For this review, take the finished solid that the model builds, in its own axes (mm). Face numbers are marked on the shaded views. A direction names the side the tool comes from. Round coordinates to 2 decimals unless told otherwise and drop trailing zeros. Loops run counter-clockwise (first coordinate to the right, second up) from the corner with the lowest first, then second, coordinate; pieces in that order, holes last.
1. Clearance check with flat-ended pins moving along their axes: pin 1 Ø2 at (x, z) = (16, 13) entering from +Y; pin 2 Ø2 at (x, y) = (14, 8.5) entering from +Z; pin 3 Ø1.8 at (x, z) = (9.5, 6) entering from +Y. State where each tip first meets the part, or that it passes through.
2. Tool access review of the marked faces 4, 5 and 6: name each direction out of +Z, -Z, +X, -X, +Y, -Y from which nothing blocks a thin tool from reaching the whole face with its end or side.
3. Consider section A-A on y = 15. State the section outline as (x, z) points, then the cut area to 3 significant figures.
4. Consider section B-B on x = 10. State the section outline as (y, z) points, then the cut area to 3 significant figures.
5. Draft analysis for pull direction X (two halves, no side actions). For the marked faces 1, 2 and 3, state which applies: released by +X, released by -X, zero draft, split by the parting line, or undercut.
6. Consider section D-D on z = 13. State the section outline as (x, y) points.
7. Consider section C-C on x = 5.25. State the section outline as (y, z) points, then the cut area to 3 significant figures.
8. To check wall thickness, follow line 1 along Y through (x, z) = (10, 2.05); line 2 along Z through (x, y) = (6.75, 8); line 3 along Z through (x, y) = (3, 17.5). State the ranges of each line that lie inside material, in increasing order.
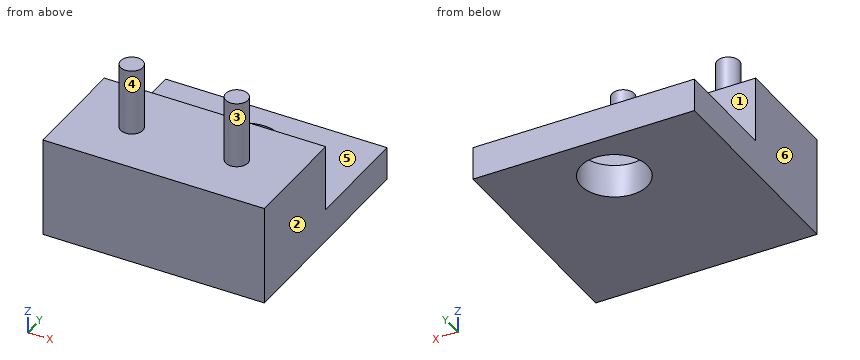
from build123d import *

# Parameters (mm, degrees)
SKETCH_1_W          = 20
SKETCH_1_H          = 20
EXTRUDE_1_DEPTH     = 9
SKETCH_2_R          = 1
EXTRUDE_2_DEPTH     = 6
SKETCH_3_W          = 20
SKETCH_3_H          = 10
CUT_EXTRUDE_1_DEPTH = 6
CUT_EXTRUDE_2_REACH = 32.725
SKETCH_4_R          = 3


with BuildPart() as part:
    # 草图1 → 凸台-拉伸1 (new body)
    with BuildSketch(Plane.XY):
        with Locations((10, 10)):
            Rectangle(SKETCH_1_W, SKETCH_1_H)
    extrude(amount=EXTRUDE_1_DEPTH)

    # 草图2 → 凸台-拉伸2 (add)
    with BuildSketch(Plane.XY.offset(9)):
        with Locations(Location((5.25, 5, 0), (0, 0, 180))):
            Circle(SKETCH_2_R)
        with Locations(Location((14.749981105, 4.981052524, 0), (0, 0, 180))):
            Circle(SKETCH_2_R)
    extrude(amount=EXTRUDE_2_DEPTH)

    # 草图3 → 切除-拉伸1 (cut)
    with BuildSketch(Plane.XY.offset(9)):
        with Locations((10, 15)):
            Rectangle(SKETCH_3_W, SKETCH_3_H)
    extrude(amount=-CUT_EXTRUDE_1_DEPTH, mode=Mode.SUBTRACT)

    # 草图4 → 切除-拉伸2 (cut, up to next)
    with BuildSketch(Plane.XY.offset(3), mode=Mode.PRIVATE) as cut_extrude_2_sk1:
        with Locations((10, 15)):
            Circle(SKETCH_4_R)
    cut_extrude_2_tool1 = extrude(cut_extrude_2_sk1.sketch, amount=-CUT_EXTRUDE_2_REACH, mode=Mode.PRIVATE) & part.part
    add(cut_extrude_2_tool1.solids().sort_by_distance((10, 15, 3))[0], mode=Mode.SUBTRACT)


solid = part.part
Resolved:
1. pin 1: stops at y = 5.95
1. pin 2: stops at z = 9
1. pin 3: stops at y = 10
2. face 4: +Z
2. face 5: +Z, +X, -X, +Y
2. face 6: +Z, -Z, -X, +Y, -Y
3. outline: (0, 0) - (7, 0) - (7, 3) - (0, 3) - close; (13, 0) - (20, 0) - (20, 3) - (13, 3) - close
3. area: 42.0 mm2
4. outline: (0, 0) - (12, 0) - (12, 3) - (10, 3) - (10, 9) - (0, 9) - close; (18, 0) - (20, 0) - (20, 3) - (18, 3) - close
4. area: 102 mm2
5. face 1: zero draft
5. face 2: released by +X
5. face 3: undercut
6. outline: circle Ø2 at (5.25, 5); circle Ø2 at (14.75, 4.98)
7. outline: (0, 0) - (20, 0) - (20, 3) - (10, 3) - (10, 9) - (6, 9) - (6, 15) - (4, 15) - (4, 9) - (0, 9) - close
7. area: 132 mm2
8. line 1: y = 0 to 12, 18 to 20
8. line 2: z = 0 to 9
8. line 3: z = 0 to 3
